Read the model definition and answer for the solid it produces. Units are mm, in the model's axes. Face numbers are marked on the shaded views. Give positions to 0.01 mm unless a question says otherwise; leave off trailing zeros. Order: outer loops, then holes, each group sorted by start corner. A loop starts at its lowest first (then second) coordinate and runs counter-clockwise, first axis right, second up.
Item 1: A cutting plane is placed at C-C (y = 16). State how many separate pieces and enclosed holes the cut face has, plus the area to 3 significant figures.
Item 2: Given pin 1 Ø4.5 at (x, y) = (-16, 16) entering from +Z, flat-ended and moving along its own axis, determine where the tip first touches the part or whether it passes through.
Item 3: The mould has two halves that part along X. Classify the marked faces 1, 2 and 3: +X half, -X half, draft (parallel to the pull), parting line (faces both ways), or undercut.
Item 4: A cutting plane is placed at B-B (z = 3.75). Write down the section's boundary in (x, y).
Item 5: Find the intervals of material crossed by line 1 along Y through (x, z) = (16, 3.5); line 2 along Y through (x, z) = (-17.5, 9.5); line 3 along Y through (x, z) = (10, 2), in increasing order.
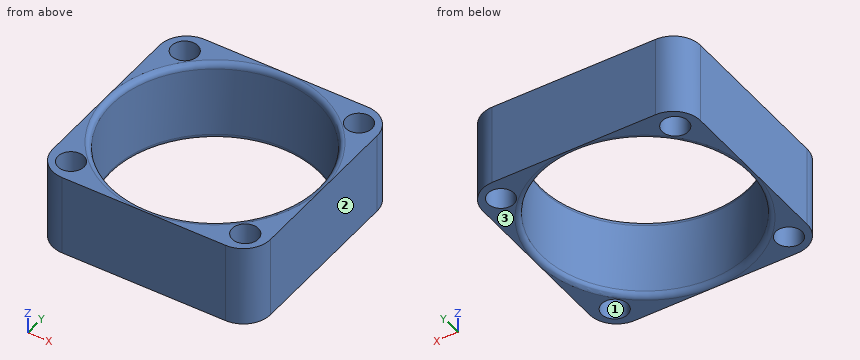
from build123d import *

# Parameters (mm, degrees)
F0_W     = 40
F0_H     = 40
F0_R     = 2.4
F0_R_2   = 19
F1_DEPTH = 15
F2_R     = 5
F3_R     = 0.99999


# Not quite as in the source:
# - a fillet or chamfer is up to 0.001 mm smaller than in the source, because OpenCascade refuses the exact size


with BuildPart() as f1:
    # F0 (on Top) → F1 (new body)
    with BuildSketch(Plane.XY):
        Rectangle(F0_W, F0_H)
        with Locations((-16, -16)):
            Circle(F0_R, mode=Mode.SUBTRACT)
        with Locations((16, -16)):
            Circle(F0_R, mode=Mode.SUBTRACT)
        with Locations((-16, 16)):
            Circle(F0_R, mode=Mode.SUBTRACT)
        Circle(F0_R_2, mode=Mode.SUBTRACT)
        with Locations((16, 16)):
            Circle(F0_R, mode=Mode.SUBTRACT)
    extrude(amount=F1_DEPTH)

    # F2
    f2_edges = [f1.edges().sort_by_distance(p)[0] for p in [
        (20, 20, 7.5),
        (20, -20, 7.5),
        (-20, 20, 7.5),
        (-20, -20, 7.5),
    ]]
    fillet(f2_edges, radius=F2_R)

    # F3 (radius 1 in the source; OpenCascade refuses exactly that, so slightly less here)
    f3_edges = [f1.edges().sort_by_distance(p)[0] for p in [
        (-19, 0, 15),
        (-19, 0, 0),
    ]]
    fillet(f3_edges, radius=F3_R)


solid = f1.part
Response values:
1. separate pieces: 4
1. enclosed holes: 0
1. area: 144 mm2
2. pin 1: passes through
3. face 1: undercut
3. face 2: +X half
3. face 3: draft
4. outline: (-20, -15) arc R5 ccw to (-15, -20) - (15, -20) arc R5 ccw to (20, -15) - (20, 15) arc R5 ccw to (15, 20) - (-15, 20) arc R5 ccw to (-20, 15) - close; hole circle Ø38 at (0, 0); hole circle Ø4.8 at (-16, -16); hole circle Ø4.8 at (-16, 16); hole circle Ø4.8 at (16, -16); hole circle Ø4.8 at (16, 16)
5. line 1: y = -19.9 to -18.4, -13.6 to -10.25, 10.25 to 13.6, 18.4 to 19.9
5. line 2: y = -19.33 to -17.87, -14.13 to -7.4, 7.4 to 14.13, 17.87 to 19.33
5. line 3: y = -20 to -16.16, 16.16 to 20
